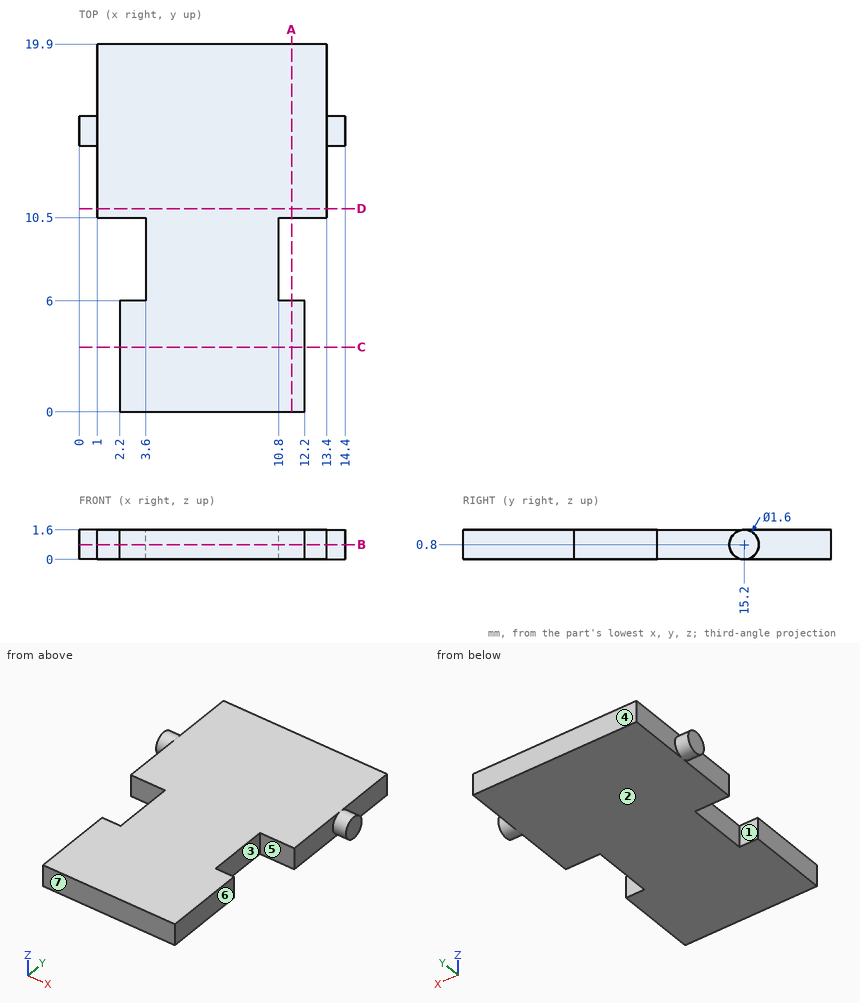
Input: dimensioned drawing with shaded views. Units: mm. Origin: part minimum x, y, z. A direction names the side the tool comes from. Coordinates: 2 decimals unless noted, no trailing zeros. Loops run counter-clockwise (first coordinate to the right, second up) from the corner with the lowest first, then second, coordinate; pieces in that order, holes last. Notation, with made-up numbers: (-6.75, 57.5) - (40.25, 57.5) arc R18 cw to (40.25, 71.5) - close; hole circle Ø5 at (84, 78). An arc over 180 degrees is marked (long way). One line per question, with ' | ' between items. Start each with the question number.
(1) Cut plane C-C on y = 3.5. Output: boundary loops of the cut face in (x, z), and give its area (3 significant figures).
(2) First-contact query: pin 1 (0.8 mm diameter, centred on y = 18.5, z = 1, fed in from -X); pin 2 (0.5 mm diameter, centred on x = 1.5, z = 1, fed in from -Y); pin 3 (0.5 mm diameter, centred on y = 8.5, z = 1, fed in from +X). Flat tips, straight axial feed; report the tip coordinate or a pass-through.
(3) Cut plane A-A on x = 11.5. Output: boundary loops of the cut face in (y, z), and give its area (3 significant figures).
(4) Draft query along Y for the marked faces 4, 5, 6 and 7. Return one class per face: +Y half, -Y half, draft (parallel to the pull), parting line (faces both ways), or undercut.
(5) Reachability of the marked faces 1, 2 and 3 from +Z, -Z, +X, -X, +Y, -Y: full face, straight path, thin tool, end or side. Return the list, or none.
(6) Cut plane D-D on y = 11. Output: boundary loops of the cut face in (x, z).
(7) Cut plane B-B on z = 0.8. Output: boundary loops of the cut face in (x, y).
(8) Ray query, L1, parallel to Y at x = 3.5, z = 0.4; L2, parallel to X at y = 12.25, z = 0.5; L3, parallel to X at y = 1.5, z = 0.25. Return the intervals inside material, ascending. Write a range as from..to.
Here are the results:
1) outline: (2.2, 0) - (12.2, 0) - (12.2, 1.6) - (2.2, 1.6) - close | area: 16.0 mm²
2) pin 1: x = 1 | pin 2: y = 10.5 | pin 3: x = 10.8
3) outline: (0, 0) - (6, 0) - (6, 1.6) - (0, 1.6) - close; (10.5, 0) - (19.9, 0) - (19.9, 1.6) - (10.5, 1.6) - close | area: 24.6 mm²
4) face 4: +Y half | face 5: undercut | face 6: draft | face 7: -Y half
5) face 1: +Z, -Z, -X | face 2: -Z, +X, -X, +Y, -Y | face 3: +Z, -Z, +X
6) outline: (1, 0) - (13.4, 0) - (13.4, 1.6) - (1, 1.6) - close
7) outline: (0, 14.4) - (1, 14.4) - (1, 10.5) - (3.6, 10.5) - (3.6, 6) - (2.2, 6) - (2.2, 0) - (12.2, 0) - (12.2, 6) - (10.8, 6) - (10.8, 10.5) - (13.4, 10.5) - (13.4, 14.4) - (14.4, 14.4) - (14.4, 16) - (13.4, 16) - (13.4, 19.9) - (1, 19.9) - (1, 16) - (0, 16) - close
8) L1: 0..6, 10.5..19.9 | L2: 1..13.4 | L3: 2.2..12.2
